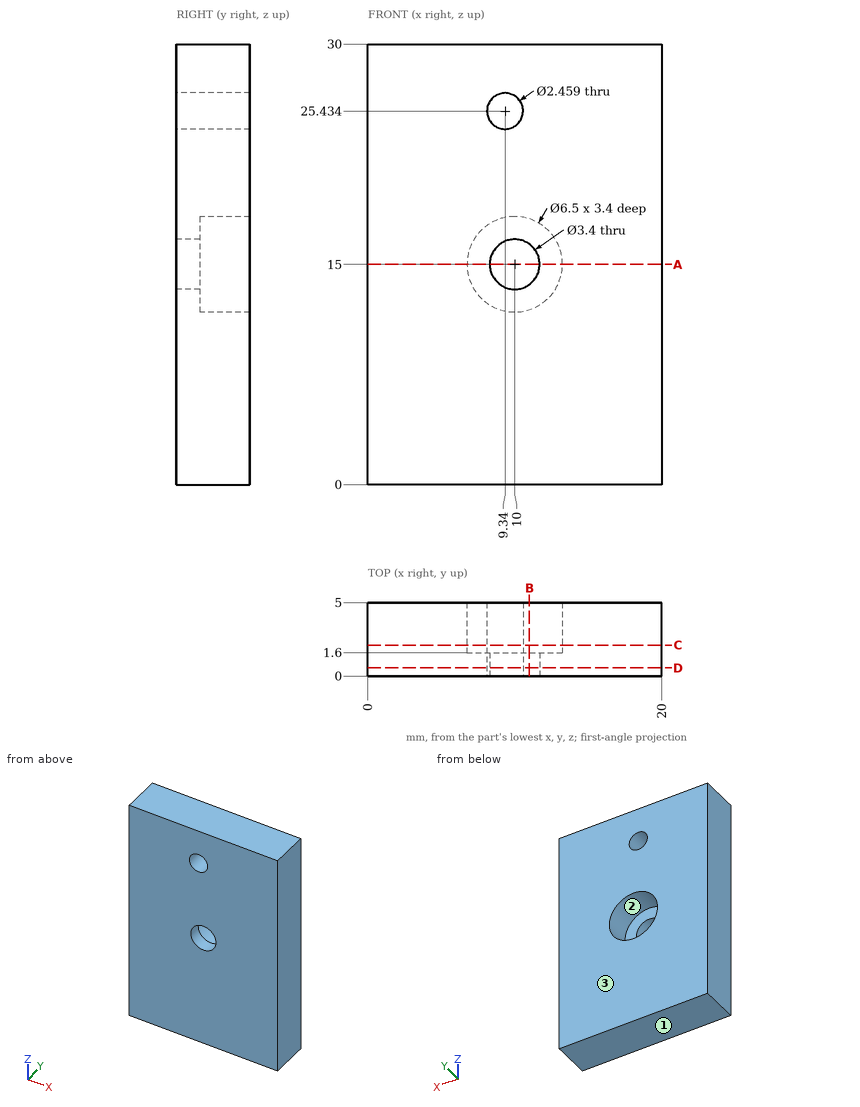
Job drawing, mm, ordinate dimensions from the low corner. One solid piece. Coordinates: 2 decimals unless noted, no trailing zeros. Write each loop counter-clockwise with the first axis right and the second up, starting at its lowest first coordinate (ties: lowest second). Pieces come first, ordered by that corner, then holes.
Item 1: Pin check, flat tips, straight feed: pin 1 (2 mm diameter, centred on x = 10, z = 15, fed in from +Y); pin 2 (5 mm diameter, centred on x = 9.5, z = 15, fed in from +Y). Stop position of each tip, or through.
Item 2: Slice it at B-B (x = 11). Write the cut outline in (y, z) (1 decimal).
Item 3: Probe line 1 (X direction, y = 4.25, z = 15); line 2 (Z direction, x = 9, y = 2); line 3 (X direction, y = 1.05, z = 15). List the from-to ranges inside material, lowest first.
Item 4: Slice it at A-A (z = 15). Write the cut outline in (x, y).
Item 5: Slice it at D-D (y = 0.55). Write the cut outline in (x, z).
Item 6: Mould opens along Z. For the marked faces 1, 2 and 3 say: released by +Z, released by -Z, zero draft, split by the parting line, or undercut.
Item 7: Slice it at C-C (y = 2.1). Write the cut outline in (x, z).
Results found:
1. pin 1: passes through
1. pin 2: stops at y = 1.6
2. outline: (0, 0) - (5, 0) - (5, 11.9) - (1.6, 11.9) - (1.6, 13.6) - (0, 13.6) - close; (0, 16.4) - (1.6, 16.4) - (1.6, 18.1) - (5, 18.1) - (5, 30) - (0, 30) - close
3. line 1: x = 0 to 6.75, 13.25 to 20
3. line 2: z = 0 to 11.91, 18.09 to 24.25, 26.62 to 30
3. line 3: x = 0 to 8.3, 11.7 to 20
4. outline: (0, 0) - (8.3, 0) - (8.3, 1.6) - (6.75, 1.6) - (6.75, 5) - (0, 5) - close; (11.7, 0) - (20, 0) - (20, 5) - (13.25, 5) - (13.25, 1.6) - (11.7, 1.6) - close
5. outline: (0, 0) - (20, 0) - (20, 30) - (0, 30) - close; hole circle Ø2.46 at (9.34, 25.43); hole circle Ø3.4 at (10, 15)
6. face 1: released by -Z
6. face 2: undercut
6. face 3: zero draft
7. outline: (0, 0) - (20, 0) - (20, 30) - (0, 30) - close; hole circle Ø6.5 at (10, 15); hole circle Ø2.46 at (9.34, 25.43)
